Read the model definition and answer for the solid it produces. Units are mm, in the model's axes. Face numbers are marked on the shaded views. Give positions to 0.01 mm unless a question says otherwise; leave off trailing zeros. Order: outer loops, then holes, each group sorted by start corner. A loop starts at its lowest first (then second) coordinate and runs counter-clockwise, first axis right, second up. Notation, with made-up numbers: M 89.25,-4.5 L 107.25,-4.5 A17 cw 107.25,17.5 Z; hole C -18.5,18.5 d9. An arc over 180 degrees is marked long. One line per item, written item: value.
from build123d import *

# Parameters (mm, degrees)
F1_W     = 132.6
F1_H     = 82.6
F1_R     = 2.25
F2_DEPTH = 4.2
F0_W     = 82.6
F0_H     = 32.6
F0_W_2   = 72.6
F0_H_2   = 22.6
F3_DEPTH = 4
F4_R     = 2.655
F5_DEPTH = 3.8
F5_TAPER = 1.6
F6_R     = 1.75
F7_DEPTH = 4.201
F8_R     = 1.99999


# Not quite as in the source:
# - a fillet or chamfer is up to 0.001 mm smaller than in the source, because OpenCascade refuses the exact size


with BuildPart() as f2:
    # F1 (on Top) → F2 (new body)
    with BuildSketch(Plane.XY):
        Rectangle(F1_W, F1_H)
        with Locations((-53.8, -28.8)):
            Circle(F1_R, mode=Mode.SUBTRACT)
        with Locations((53.8, -28.8)):
            Circle(F1_R, mode=Mode.SUBTRACT)
        with Locations((-53.8, 28.8)):
            Circle(F1_R, mode=Mode.SUBTRACT)
        with Locations((53.8, 28.8)):
            Circle(F1_R, mode=Mode.SUBTRACT)
    extrude(amount=-F2_DEPTH)

    # F0 (on Top) → F3 (join)
    with BuildSketch(Plane.XY):
        Rectangle(F0_W, F0_H)
        Rectangle(F0_W_2, F0_H_2, mode=Mode.SUBTRACT)
    extrude(amount=F3_DEPTH)

    # F4 (on face) → F5 (cut)
    with BuildSketch(Plane.XY):
        with Locations((-31, 0)):
            Circle(F4_R)
        with Locations((31, 0)):
            Circle(F4_R)
    extrude(amount=-F5_DEPTH, taper=F5_TAPER, mode=Mode.SUBTRACT)

    # F6 (on face) → F7 (cut, through all)
    with BuildSketch(Plane.XY):
        with Locations((31, 0)):
            Circle(F6_R)
        with Locations((-31, 0)):
            Circle(F6_R)
    extrude(amount=-F7_DEPTH, mode=Mode.SUBTRACT)

    # F8 (radius 2 in the source; OpenCascade refuses exactly that, so slightly less here)
    f8_edges = [f2.edges().sort_by_distance(p)[0] for p in [
        (0, 16.3, 0),
        (-41.3, 0, 0),
        (0, -16.3, 0),
        (41.3, 0, 0),
        (0, -16.3, 4),
        (41.3, 0, 4),
        (0, 16.3, 4),
        (-41.3, 0, 4),
    ]]
    fillet(f8_edges, radius=F8_R)


solid = f2.part
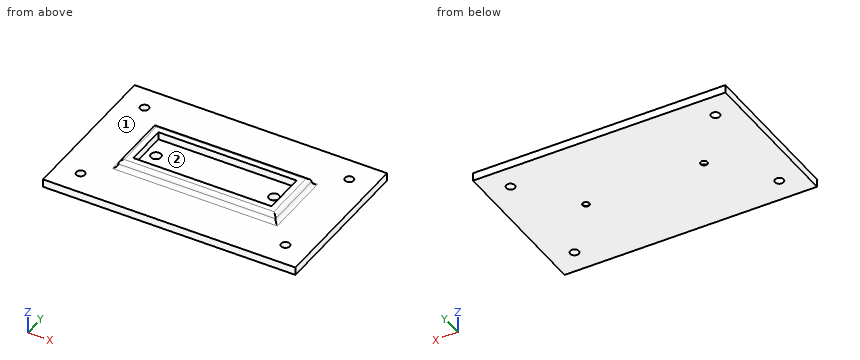
1) Find section B-B, the plane y = -28.8. Write down the section's boundary in (x, z), plus the area to 3 significant figures.
Reported:
outline: M -66.3,-4.2 L -56.05,-4.2 L -56.05,0 L -66.3,0 Z; M -51.55,-4.2 L 51.55,-4.2 L 51.55,0 L -51.55,0 Z; M 56.05,-4.2 L 66.3,-4.2 L 66.3,0 L 56.05,0 Z
area: 519 mm^2
2) Consider probe 1 along Y at (x, z) = (-53.8, -2.35); probe 2 along Y at (x, z) = (31, -4); probe 3 along Y at (x, z) = (-16.5, 2.25). Determine where each line is inside the solid, lowest interval first.
Reported:
probe 1: y = -41.3 to -31.05, -26.55 to 26.55, 31.05 to 41.3
probe 2: y = -41.3 to -1.75, 1.75 to 41.3
probe 3: y = -16.28 to -11.3, 11.3 to 16.28
3) Each of these flat-tipped pins is pushed along its axis until it touches: pin 1 Ø2.5 at (x, y) = (53.8, 28.8) entering from -Z; pin 2 Ø1 at (x, z) = (27, 2.5) entering from -Y; pin 3 Ø8 at (x, y) = (44, -26) entering from +Z; pin 4 Ø2.5 at (x, y) = (30.5, -0.5) entering from +Z. Where does it stop, or does it pass through?
Reported:
pin 1: passes through
pin 2: stops at y = -16.3
pin 3: stops at z = 0
pin 4: stops at z = -3.8
4) Find section A-A, the plane x = -53.8. Write down the section's boundary in (y, z).
Reported:
outline: M -41.3,-4.2 L -31.05,-4.2 L -31.05,0 L -41.3,0 Z; M -26.55,-4.2 L 26.55,-4.2 L 26.55,0 L -26.55,0 Z; M 31.05,-4.2 L 41.3,-4.2 L 41.3,0 L 31.05,0 Z
5) Determine the mould class of the marked faces 1 and 2 for opening direction Y: +Y half, -Y half, draft (parallel to the pull), parting line (faces both ways), or undercut.
Reported:
face 1: draft
face 2: undercut
